The model under review builds one solid part; all positions refer to its coordinate system, in mm. Coordinates: 2 decimals unless noted, no trailing zeros. Write each loop counter-clockwise with the first axis right and the second up, starting at its lowest first coordinate (ties: lowest second). Pieces come first, ordered by that corner, then holes.
```python
from build123d import *

# Parameters (mm, degrees)
F0_R     = 2.5
F1_DEPTH = 10
F2_DEPTH = 5
F3_R     = 5


with BuildPart() as f1:
    # F0 (on Top) → F1 (new body)
    with BuildSketch(Plane.XY):
        with BuildLine():
            ThreePointArc((-105.3399322968, 31.6780470312), (-107.7412608362, 22.1770312131), (-109.287464972, 12.5))
            ThreePointArc((-109.287464972, 12.5), (-110, 0), (-109.287464972, -12.5))
            ThreePointArc((-109.287464972, -12.5), (-107.5911875881, -22.8940244035), (-104.9086893631, -33.0781936646))
            Line((-104.9086893631, -33.0781936646), (-96, -33.0781936646))
            Line((-96, -33.0781936646), (-96, 31.6780470312))
            Line((-96, 31.6780470312), (-105.3399322968, 31.6780470312))
        make_face()
        with Locations((-102.7974784374, 0)):
            Circle(F0_R, mode=Mode.SUBTRACT)
    extrude(amount=F1_DEPTH)

    # F0 (on Top) → F2 (join)
    with BuildSketch(Plane.XY):
        with BuildLine():
            Line((-110, 12.5), (-109.287464972, 12.5))
            ThreePointArc((-109.287464972, 12.5), (-107.7412608362, 22.1770312131), (-105.3399322968, 31.6780470312))
            Line((-105.3399322968, 31.6780470312), (-126, 31.6780470312))
            Line((-126, 31.6780470312), (-126, 12.5))
            Line((-126, 12.5), (-110, 12.5))
        make_face()
        with BuildLine():
            ThreePointArc((-109.287464972, -12.5), (-110, 0), (-109.287464972, 12.5))
            Line((-109.287464972, 12.5), (-110, 12.5))
            Line((-110, 12.5), (-126, 12.5))
            Line((-126, 12.5), (-126, -12.5))
            Line((-126, -12.5), (-110, -12.5))
            Line((-110, -12.5), (-109.287464972, -12.5))
        make_face()
        with BuildLine():
            ThreePointArc((-104.9086893631, -33.0781936646), (-107.5911875881, -22.8940244035), (-109.287464972, -12.5))
            Line((-109.287464972, -12.5), (-110, -12.5))
            Line((-110, -12.5), (-126, -12.5))
            Line((-126, -12.5), (-126, -33.0781936646))
            Line((-126, -33.0781936646), (-104.9086893631, -33.0781936646))
        make_face()
    extrude(amount=F2_DEPTH)

    # F3
    f3_edges = [f1.edges().sort_by_distance(p)[0] for p in [
        (-126, -33.078194, 2.5),
        (-96, -33.078194, 5),
        (-126, 31.678047, 2.5),
        (-96, 31.678047, 5),
    ]]
    fillet(f3_edges, radius=F3_R)


solid = f1.part
```
Item 1: Take a section at C-C, the plane x = -111. Write out the cut boundary in (y, z).
Solved:
outline: (-33.08, 0) - (31.68, 0) - (31.68, 5) - (-33.08, 5) - close
Item 2: Take a section at A-A, the plane y = 0. Write out the cut boundary in (x, z).
Solved:
outline: (-126, 0) - (-105.3, 0) - (-105.3, 10) - (-110, 10) - (-110, 5) - (-126, 5) - close; (-100.3, 0) - (-96, 0) - (-96, 10) - (-100.3, 10) - close
Item 3: Mouldability with a two-part tool opening along X and no side actions: class faces 1 (the face through (-105.295, 0.11, 4.93)), 2 (the face through (-97.5, 30.25, 5.07)), 3 (the face through (-109, 31.678, 4)), 4 (the face through (-124.5, -31.65, 2.54)) as pulls with the +X half, pulls with the -X half, needs draft (parallel to the pull), parting line crosses it, or undercut.
Solved:
face 1: undercut
face 2: pulls with the +X half
face 3: needs draft
face 4: pulls with the -X half
Item 4: For pin 1 (8 mm diameter, centred on x = -123, y = -12.5, fed in from +Z), flat-tipped, find the tip position at first contact; note if it passes through.
Solved:
pin 1: stops at z = 5
Item 5: Take a section at D-D, the plane z = 1.5. Write out the cut boundary in (x, y).
Solved:
outline: (-126, -28.08) arc R5 ccw to (-121, -33.08) - (-101, -33.08) arc R5 ccw to (-96, -28.08) - (-96, 26.68) arc R5 ccw to (-101, 31.68) - (-121, 31.68) arc R5 ccw to (-126, 26.68) - close; hole circle Ø5 at (-102.8, 0)
Item 6: Take a section at B-B, the plane z = 5.75. Write out the cut boundary in (x, y).
Solved:
outline: (-105.34, 31.68) arc R110 ccw to (-104.91, -33.08) - (-101, -33.08) arc R5 ccw to (-96, -28.08) - (-96, 26.68) arc R5 ccw to (-101, 31.68) - close; hole circle Ø5 at (-102.8, 0)
Item 7: To check wall thickness, follow line 1 along Z through (x, y) = (-111, -8); line 2 along Y through (x, z) = (-100.5, 5.25); line 3 along Y through (x, z) = (-103.25, 5.5). State the ranges of each line that lie inside material, in increasing order.
Solved:
line 1: z = 0 to 5
line 2: y = -33.05 to -0.99, 0.99 to 31.65
line 3: y = -33.08 to -2.46, 2.46 to 31.68
